Could you check a few things on this model? Use its own coordinates, in mm. Give positions to 0.01 mm unless a question says otherwise; leave off trailing zeros. Order: outer loops, then holes, each group sorted by start corner. A loop starts at its lowest first (then second) coordinate and runs counter-clockwise, first axis right, second up. Notation, with made-up numbers: (49.5, -19) -> (65.5, -19) arc R23 ccw to (65.5, 10) -> close; hole circle Ø5 at (70.25, 18.5). An arc over 180 degrees is marked (long way). One line per item, written item: value.
```python
from build123d import *

# Parameters (mm, degrees)
F0_W     = 52
F0_H     = 50.8
F1_DEPTH = 5
F3_DEPTH = 52
F5_D     = 3.302
F6_R     = 24
F7_DEPTH = 32.036534


with BuildPart() as f1:
    # F0 (on Front) → F1 (new body)
    with BuildSketch(Plane.XZ):
        with Locations((26, 25.4)):
            Rectangle(F0_W, F0_H)
    extrude(amount=F1_DEPTH)

    # F2 (on face) → F3 (join, through all)
    with BuildSketch(Plane(origin=(0, 0, 0), x_dir=(0, -1, 0), z_dir=(-1, 0, 0))):
        Polygon((5, 0), (0, 0), (38.234019, -38.234019), (41.769553, -34.698485), (5, 2.071068), align=None)
    extrude(amount=-F3_DEPTH)

    # F5 (through all)
    with Locations(Plane(origin=(0, -3.535534, 3.535534), x_dir=(1, 0, 0), z_dir=(0, -0.707107, 0.707107))):
        with Locations((48.5, -5.571068), (48.5, -50.571068), (3.5, -50.571068), (3.5, -5.571068)):
            Hole(F5_D / 2)

    # F6 (on face) → F7 (cut, through all)
    with BuildSketch(Plane(origin=(0, -3.535534, 3.535534), x_dir=(1, 0, 0), z_dir=(0, -0.707107, 0.707107))):
        with Locations((26, -28.071068)):
            Circle(F6_R)
    extrude(amount=-F7_DEPTH, mode=Mode.SUBTRACT)


solid = f1.part
```
1) If I drill on line 1 along Y through (x, z) = (43.5, 27); line 2 along X through (y, z) = (-36, -33); line 3 along X through (y, z) = (-16, -13), over which ranges is the centre line in solid material (lowest first)?
Answer below:
line 1: y = -5 to 0
line 2: x = 0 to 13.89, 38.11 to 52
line 3: x = 0 to 3.22, 48.78 to 52
2) Suppose I cut it at D-D, the plane x = 15.5. Write out the boundary of the cut face in (y, z), then the cut area to 3 significant figures.
Answer below:
outline: (-41.77, -34.7) -> (-38.23, -38.23) -> (-35.11, -35.11) -> (-38.65, -31.57) -> close; (-8.12, -1.05) -> (-4.59, -4.59) -> (0, 0) -> (0, 50.8) -> (-5, 50.8) -> (-5, 2.07) -> close
area: 298 mm2
3) We'd pull the mould along Y, two halves only. Please class faces 1 (the flat face through (26, -2, 50.8)), 2 (the cylindrical face through (47.74, -38.54, -35.05)), 3 (the cylindrical face through (2.74, -38.54, -35.05)), 4 (the flat face through (26, -5, 27)): +Y half, -Y half, draft (parallel to the pull), parting line (faces both ways), or undercut.
Answer below:
face 1: draft
face 2: undercut
face 3: undercut
face 4: -Y half
4) For P1, Ø6, axis at x = 29, y = -11.5, coming from the +Z side; P2, Ø24.5, axis at x = 33.5, z = 20.5, coming from the -Y side; P3, Ø6, axis at x = 27, z = 1, coming from the -Y side (3 decimals); P4, Ø3, axis at x = 41.5, y = -36.5, coming from the -Z side, each with a flat end and sliding along its axis, tell me the tip position at first contact or that it passes through.
Answer below:
P1: passes through
P2: stops at y = -5
P3: stops at y = -6.645
P4: stops at z = -38
5) Suppose I cut it at A-A, the plane x = 39. Write out the boundary of the cut face in (y, z).
Answer below:
outline: (-41.77, -34.7) -> (-38.23, -38.23) -> (-34.11, -34.11) -> (-37.65, -30.58) -> close; (-9.12, -2.05) -> (-5.58, -5.58) -> (0, 0) -> (0, 50.8) -> (-5, 50.8) -> (-5, 2.07) -> close
6) Suppose I cut it at B-B, the plane x = 48. Write out the boundary of the cut face in (y, z), then the cut area to 3 significant figures.
Answer below:
outline: (-41.77, -34.7) -> (-38.23, -38.23) -> (-36.87, -36.87) -> (-40.41, -33.34) -> close; (-38.18, -31.11) -> (-34.65, -34.65) -> (-26.63, -26.63) -> (-30.17, -23.1) -> close; (-16.6, -9.53) -> (-13.07, -13.07) -> (-5.05, -5.05) -> (-8.59, -1.52) -> close; (-6.36, 0.71) -> (-2.83, -2.83) -> (0, 0) -> (0, 50.8) -> (-5, 50.8) -> (-5, 2.07) -> close
area: 387 mm2
7) Suppose I cut it at C-C, the plane z = 37.5. Write out the boundary of the cut face in (x, y), then the cut area to 3 significant figures.
Answer below:
outline: (0, -5) -> (52, -5) -> (52, 0) -> (0, 0) -> close
area: 260 mm2
